The drawing under review shows one solid part. Ordinate dimensions are in mm from its lowest x, y, z. Coordinates: 2 decimals unless noted, no trailing zeros. Write each loop counter-clockwise with the first axis right and the second up, starting at its lowest first coordinate (ties: lowest second). Pieces come first, ordered by that corner, then holes. Notation, with made-up numbers: (28.25, 50.5) -> (45.25, 50.5) arc R17 cw to (45.25, 78.5) -> close; hole circle Ø9 at (-35.75, -24). An arc over 180 degrees is marked (long way). Put each result on its own line as item: value. Start each with the question number.
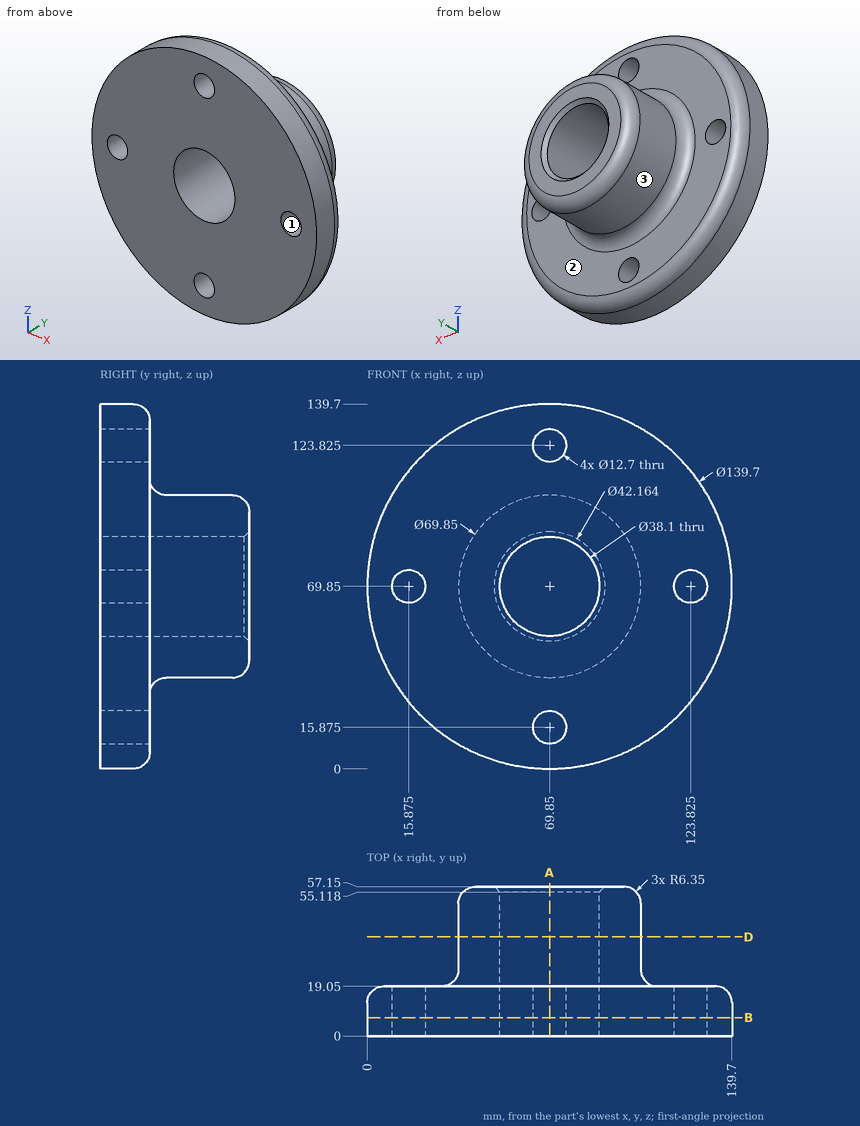
1. The part is to be moulded in two halves that separate along Z. For the marked faces 1, 2 and 3, say which applies: released by +Z, released by -Z, zero draft, split by the parting line, or undercut.
2. Consider section A-A on x = 69.85. State how many separate pieces and enclosed holes the cut face has, then the cut area to 3 significant figures.
3. Consider section D-D on y = 38. State the section outline as (x, z) points (3 decimals).
4. Consider section B-B on y = 7. State the section outline as (x, z) points (3 decimals), then the cut area to 3 significant figures.
5. Insertion check: P1, Ø23, axis at x = 69.85, z = 69.85, coming from the -Y side; P2, Ø4, axis at x = 112.5, z = 34.5, coming from the +Y side; P3, Ø4, axis at y = 22.5, z = 80, coming from the +X side; P4, Ø16.5, axis at x = 69.85, z = 123.825, coming from the -Y side. Each pin has a flat end and moves straight along its axis. Give the tip position at first contact, or say it passes through.
6. Wall thickness on line 1 (Z direction, x = 69, y = 7); line 2 (Z direction, x = 124, y = 16); line 3 (Y direction, x = 114.5, z = 55): over which ranges is each line inside the solid? List them lowest first. Write a range as from..to.
Output values:
1. face 1: undercut
1. face 2: zero draft
1. face 3: split by the parting line
2. separate pieces: 4
2. enclosed holes: 0
2. area: 2,640 mm^2
3. outline: circle Ø69.85 at (69.85, 69.85); hole circle Ø38.1 at (69.85, 69.85)
4. outline: circle Ø139.7 at (69.85, 69.85); hole circle Ø12.7 at (15.875, 69.85); hole circle Ø38.1 at (69.85, 69.85); hole circle Ø12.7 at (69.85, 15.875); hole circle Ø12.7 at (69.85, 123.825); hole circle Ø12.7 at (123.825, 69.85)
4. area: 13,700 mm^2
5. P1: passes through
5. P2: stops at y = 19.05
5. P3: stops at x = 105.74
5. P4: stops at y = 0
6. line 1: z = 0.01..9.58, 22.17..50.82, 88.88..117.53, 130.12..139.69
6. line 2: z = 27.21..63.5, 76.2..112.49
6. line 3: y = 0..19.05
